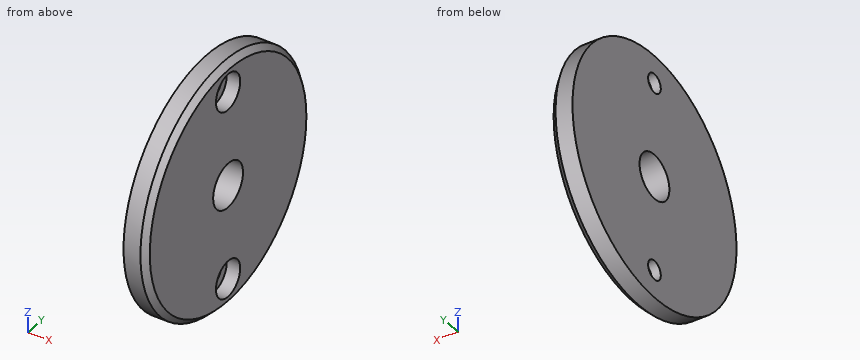
Autodesk Inventor part; units mm, degrees
ref_plane "YZ Plane" through (0, 0, 0) normal (1, 0, 0) x (0, 1, 0)
ref_plane "XZ Plane" through (0, 0, 0) normal (0, 1, 0) x (-1, 0, 0)
ref_plane "XY Plane" through (0, 0, 0) normal (0, 0, 1) x (1, 0, 0)
sketch "Sketch1" plane through (0, 0, 0) normal (1, 0, 0) x (0, 1, 0)
  circle A0 centre (0, 0) radius 22
  dimension "d0" = 44
extrude "Extrusion1" add sketch "Sketch1" along normal blind 4
sketch "Sketch2" plane through (4, 0, 0) normal (1, 0, 0) x (0, 0, -1)
  circle A0 centre (-17, 0) radius 1.5
  circle A1 centre (17, 0) radius 1.5
  point P0 (0, 0)
  dimension "d3" = 3
  dimension "d4" = 3
  dimension "d5" = 34
  dimension "d6" = 17
hole "Hole1" at (4, 0, 17) at (4, 0, -17) direction (-1, 0, 0) diameter 3.4 depth 8.8 tip angle 118 counterbore diameter 6.5 counterbore depth 2.4
sketch "Sketch3" plane through (4, 0, 0) normal (1, 0, 0) x (0, 0, -1)
  circle A0 centre (0, 0) radius 4
  dimension "d14" = 8
extrude "Extrusion2" cut sketch "Sketch3" against normal blind 4
chamfer "Chamfer1" distance 1 angle 45 1 edges at (4, -22, 0)
properties part number "kołmierz"
Geometry: final body of the model. Coordinates: model frame, mm. Round coordinates to 2 decimals unless told otherwise and drop trailing zeros. Loops run counter-clockwise (first coordinate to the right, second up) from the corner with the lowest first, then second, coordinate; pieces in that order, holes last. Notation, with made-up numbers: M 44,53 L 72,53 A11 ccw 72,59 Z; hole C 23,-18 d10. An arc over 180 degrees is marked long. One line per question, with ' | ' between items.
(1) Cut plane C-C on x = 2.45. Return the cut outline in (y, z).
Check result:
outline: C 0,0 d44; hole C 0,0 d8; hole C 0,-17 d6.5; hole C 0,17 d6.5
(2) Cut plane B-B on y = 0. Return the cut outline in (x, z).
Check result:
outline: M 0,-22 L 3,-22 L 4,-21 L 4,-20.25 L 1.6,-20.25 L 1.6,-18.7 L 0,-18.7 Z; M 0,-15.3 L 1.6,-15.3 L 1.6,-13.75 L 4,-13.75 L 4,-4 L 0,-4 Z; M 0,4 L 4,4 L 4,13.75 L 1.6,13.75 L 1.6,15.3 L 0,15.3 Z; M 0,18.7 L 1.6,18.7 L 1.6,20.25 L 4,20.25 L 4,21 L 3,22 L 0,22 Z
(3) Contact query for flat-ended pins moving along their axis: P1, Ø2, axis at y = 0, z = -15.5, coming from the +X side; P2, Ø1.5, axis at x = 1.5, y = 11, coming from the +Z side; P3, Ø1, axis at x = 0.5, z = -2, coming from the -Y side. Output: stop coordinate, or through.
Check result:
P1: stops at x = 1.6 | P2: stops at z = 19.47 | P3: stops at y = -21.95
(4) Material intervals for line 1 along Z through (x, y) = (3.6, 2); line 2 along Y through (x, z) = (2.8, -0.5); line 3 along Y through (x, z) = (1.7, -18), sorted ascending. Write a range as from..to.
Check result:
line 1: z = -21.31..-19.56, -14.44..-3.46, 3.46..14.44, 19.56..21.31 | line 2: y = -21.99..-3.97, 3.97..21.99 | line 3: y = -12.65..-3.09, 3.09..12.65
(5) Cut plane A-A on z = 0. Return the cut outline in (x, y).
Check result:
outline: M 0,-22 L 3,-22 L 4,-21 L 4,-4 L 0,-4 Z; M 0,4 L 4,4 L 4,21 L 3,22 L 0,22 Z
